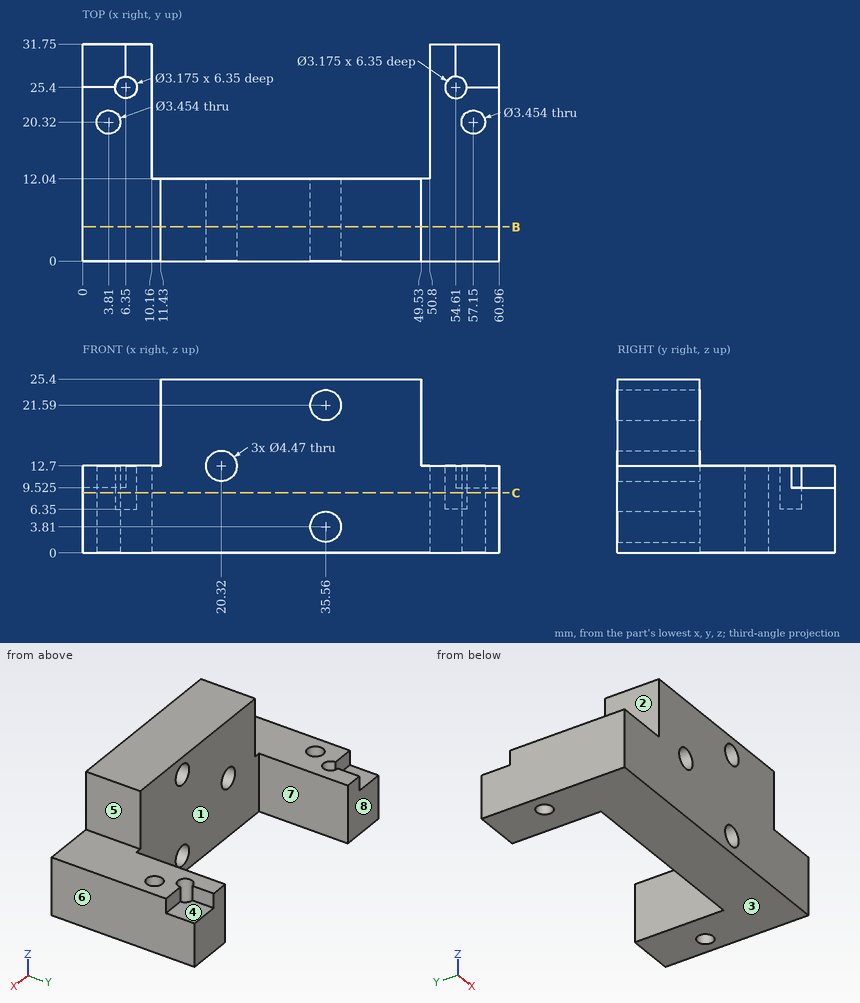
Part print with two shaded views. Sizes in mm from the minimum x, y, z corner. A direction names the side the tool comes from. Coordinates: 2 decimals unless noted, no trailing zeros. Write each loop counter-clockwise with the first axis right and the second up, starting at its lowest first coordinate (ties: lowest second). Pieces come first, ordered by that corner, then holes.
(1) Cut at B-B on y = 5. List the corners of the cut face in (x, z) (1 decimal).
(2) Pin check, flat tips, straight feed: pin 1 Ø5 at (x, y) = (59, 29) entering from +Z (3 decimals); pin 2 Ø8 at (x, z) = (21, 18) entering from +Y; pin 3 Ø7 at (x, z) = (35.56, 3.81) entering from -Y; pin 4 Ø1.6 at (x, z) = (3, 11) entering from +Y. Stop position of each tip, or through.
(3) Mould opens along X. For the marked faces 6, 7 and 8 say: pulls with the +X half, pulls with the -X half, needs draft (parallel to the pull), parting line crosses it, or undercut.
(4) Drill centre lines: line 1 (Y direction, x = 57.15, z = 8.25); line 2 (X direction, y = 25.4, z = 7.5); line 3 (Z direction, x = 35.56, y = 7.25) (1 decimal). Where is each one in solid material? Low to high.
(5) Cut at C-C on z = 8.75. State how many separate pieces and enclosed holes the cut face has, and give its area (3 significant figures).
(6) 3-axis set-ups, long thin cutter, end or side, ignore diameter. For the marked faces 1, 2, 3, 4 and 5: which of +Z, -Z, +X, -X, +Y, -Y reach the whole face in a straight line?
Working result:
1. outline: (0, 0) - (61, 0) - (61, 12.7) - (49.5, 12.7) - (49.5, 25.4) - (11.4, 25.4) - (11.4, 12.7) - (0, 12.7) - close; hole circle Ø4.5 at (20.3, 12.7); hole circle Ø4.5 at (35.6, 3.8); hole circle Ø4.5 at (35.6, 21.6)
2. pin 1: stops at z = 9.525
2. pin 2: stops at y = 12.04
2. pin 3: stops at y = 0
2. pin 4: stops at y = 25.4
3. face 6: pulls with the +X half
3. face 7: undercut
3. face 8: needs draft
4. line 1: y = 0 to 18.59, 22.05 to 31.75
4. line 2: x = 0 to 4.76, 7.94 to 10.16, 50.8 to 53.02, 56.2 to 60.96
4. line 3: z = 0 to 1.6, 6 to 19.4, 23.8 to 25.4
5. separate pieces: 1
5. enclosed holes: 4
5. area: 1,100 mm2
6. face 1: +Z, -Z, +Y
6. face 2: +Z, -X, +Y, -Y
6. face 3: -Z, +X, -X, +Y, -Y
6. face 4: +Z, +X, +Y
6. face 5: +Z, +X, +Y, -Y
